from build123d import *

# Parameters (mm, degrees)
SKETCH_1_W          = 30
SKETCH_1_H          = 20
EXTRUDE_1_DEPTH     = 10
SKETCH_2_R          = 12
CUT_EXTRUDE_1_DEPTH = 8
SKETCH_3_R          = 11
CUT_EXTRUDE_2_DEPTH = 10
CHAMFER_1_SIZE      = 1


with BuildPart() as part:
    # 스케치1 → 보스-돌출1 (new, symmetric)
    with BuildSketch(Plane.XY):
        Rectangle(SKETCH_1_W, SKETCH_1_H)
    extrude(amount=EXTRUDE_1_DEPTH, both=True)

    # 스케치2 → 컷-돌출1 (cut)
    with BuildSketch(Plane.XY.offset(10)):
        with Locations((0, 10)):
            Circle(SKETCH_2_R)
    cut_extrude_1 = extrude(amount=-CUT_EXTRUDE_1_DEPTH, mode=Mode.SUBTRACT)

    # 대칭 복사1: 컷-돌출1 across plane
    add(cut_extrude_1.mirror(Plane.XY), mode=Mode.SUBTRACT)

    # 스케치3 → 컷-돌출2 (cut)
    with BuildSketch(Plane.XY.offset(2)):
        with Locations((0, 10)):
            Circle(SKETCH_3_R)
    extrude(amount=-CUT_EXTRUDE_2_DEPTH, mode=Mode.SUBTRACT)

    # 모따기1
    chamfer_1_edges = [part.edges().sort_by_distance(p)[0] for p in [
        (0, -2, 10),
        (0, -2, -10),
    ]]
    chamfer(chamfer_1_edges, length=CHAMFER_1_SIZE)


solid = part.part
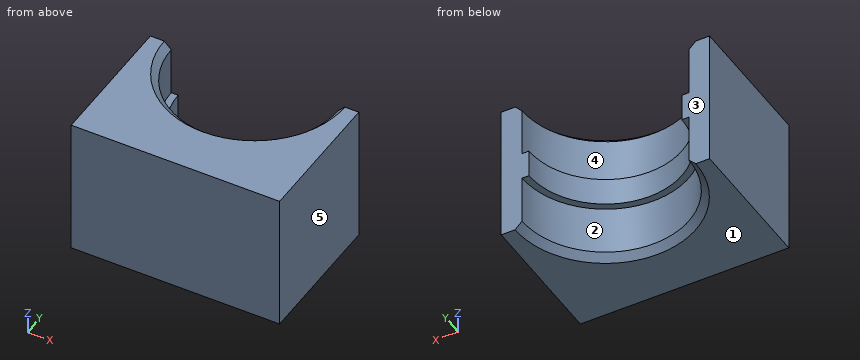
Could you check a few things on this model? Use its own coordinates, in mm. Face numbers are marked on the shaded views. A direction names the side the tool comes from. Round coordinates to 2 decimals unless told otherwise and drop trailing zeros. Write each loop counter-clockwise with the first axis right and the second up, starting at its lowest first coordinate (ties: lowest second). Pieces come first, ordered by that corner, then holes. Notation, with made-up numbers: (72, -14) -> (114, -14) arc R6 cw to (114, -3) -> close; hole circle Ø6 at (31.25, 38.5). An arc over 180 degrees is marked (long way). Use a Markdown table: item, result.
1. If we section it at C-C (z = 0): List the corners of the cut face in (x, y) for me, then the cut area to 3 significant figures.
Answer key:
| item | result |
|---|---|
| outline | (-15, -10) -> (15, -10) -> (15, 10) -> (11, 10) arc R11 cw to (-11, 10) -> (-15, 10) -> close |
| area | 410 mm^2 |
2. We'd pull the mould along X, two halves only. Please class the marked faces 3, 4 and 5: +X half, -X half, draft (parallel to the pull), parting line (faces both ways), or undercut.
Answer key:
| item | result |
|---|---|
| face 3 | draft |
| face 4 | undercut |
| face 5 | +X half |
3. If we section it at B-B (z = 7): List the corners of the cut face in (x, y) for me.
Answer key:
| item | result |
|---|---|
| outline | (-15, -10) -> (15, -10) -> (15, 10) -> (12, 10) arc R12 cw to (-12, 10) -> (-15, 10) -> close |
4. Please list where these lines run through material, in increasing order: probe 1 along X at (y, z) = (0.25, 7.5); probe 2 along X at (y, z) = (5.5, -7.25); probe 3 along Y at (x, z) = (7, -0.75).
Answer key:
| item | result |
|---|---|
| probe 1 | x = -15 to -7, 7 to 15 |
| probe 2 | x = -15 to -11.12, 11.12 to 15 |
| probe 3 | y = -10 to 1.51 |
5. Which directions (+Z, -Z, +X, -X, +Y, -Y) give clear straight access to the entire face, cutting with the end or side of a thin tool? Please do the marked faces 1 and 2.
Answer key:
| item | result |
|---|---|
| face 1 | -Z, +X, -X, +Y, -Y |
| face 2 | -Z, +Y |
6. If we section it at A-A (x = 0): List the corners of the cut face in (y, z) for me, then the cut area to 3 significant figures.
Answer key:
| item | result |
|---|---|
| outline | (-10, -10) -> (-3, -10) -> (-2, -9) -> (-2, -2) -> (-1, -2) -> (-1, 2) -> (-2, 2) -> (-2, 9) -> (-3, 10) -> (-10, 10) -> close |
| area | 163 mm^2 |
7. For pin 1 Ø9.5 at (x, y) = (4.5, 5) entering from -Z; pin 2 Ø1.5 at (x, z) = (-5.5, -3) entering from +Y; pin 3 Ø6 at (x, y) = (5.5, 3.5) entering from +Z, each with a flat end and sliding along its axis, tell me the tip position at first contact or that it passes through.
Answer key:
| item | result |
|---|---|
| pin 1 | stops at z = -2 |
| pin 2 | stops at y = -0.24 |
| pin 3 | stops at z = 2 |
